Geometry check sheet. Reference: the model listing, model coordinates, mm. A direction names the side the tool comes from. Round coordinates to 2 decimals unless told otherwise and drop trailing zeros. Order: outer loops, then holes, each group sorted by start corner. A loop starts at its lowest first (then second) coordinate and runs counter-clockwise, first axis right, second up. Notation, with made-up numbers: (83, 59) - (120, 59) arc R7 cw to (120, 66) - close; hole circle Ø3 at (-9, 49). An arc over 180 degrees is marked (long way). Use a Markdown table: item, result. Add a question column.
(1) Thickness scan on line 1 along Z through (x, y) = (12.25, -9.5); line 2 along Y through (x, z) = (6, 10.25); line 3 along X through (y, z) = (9, 3.75). Record the ranges inside material, lowest first. Write a range as [from, to].
(2) Access from +Z, -Z, +X, -X, +Y, -Y to the whole of each face (thin tool, end or side, straight path). Record for faces 4 (the face through (8.3, -22, 0.5)), 5 (the face through (0, 16.5, 7)), 6 (the face through (12, 0, 3.54)).
(3) Mould release check, pull along Z, two halves, no side actions. Record for faces 1 (the face through (12.085, -12.692, 8.977)), 2 (the face through (0, 20, 1)), 3 (the face through (13.2, 0, 9)): released by +Z, released by -Z, zero draft, split by the parting line, or undercut.
(4) Section check D-D on z = 9. Record the boundary of the cut face in (x, y).
(5) Section check A-A on x = 11.75. Record the boundary of the cut face in (y, z).
(6) Section check B-B on y = 7.5. Record the boundary of the cut face in (x, z), then the cut area to 3 significant figures.
(7) Gauge pin test, flat ends, axial feed: P1, Ø1.8, axis at x = 12.5, y = -5, coming from the +Z side; P2, Ø4, axis at y = -18.5, z = 2, coming from the +X side; P3, Ø3.5, axis at x = -5.5, z = 5.5, coming from the +Y side. Record the tip position at first contact, or that the pin passes through.
(8) Section check C-C on x = 7.5. Record the boundary of the cut face in (y, z), then the cut area to 3 significant figures.
```python
from build123d import *

# Parameters (mm, degrees)
SKETCH_1_W          = 22
SKETCH_1_H          = 53
EXTRUDE_1_DEPTH     = 1
CUT_EXTRUDE_1_DEPTH = 29.70975444
SKETCH_3_W          = 22
SKETCH_3_H          = 33
EXTRUDE_2_DEPTH     = 12
EXTRUDE_3_DEPTH     = 2.2
CHAMFER_1_SIZE      = 7
FILLET_1_R          = 5


with BuildPart() as part:
    # 草图1 → 凸台-拉伸1 (new body)
    with BuildSketch(Plane.XY):
        Rectangle(SKETCH_1_W, SKETCH_1_H)
    extrude(amount=EXTRUDE_1_DEPTH)

    # 草图2 → 切除-拉伸1 (cut, through all)
    with BuildSketch(Plane.XY.offset(1)):
        with BuildLine():
            Line((1.5, 24), (6.3, 24))
            ThreePointArc((6.3, 24), (8.3, 22), (6.3, 20))
            Line((6.3, 20), (1.5, 20))
            ThreePointArc((1.5, 20), (-0.5, 22), (1.5, 24))
        make_face()
    cut_extrude_1 = extrude(amount=-CUT_EXTRUDE_1_DEPTH, mode=Mode.SUBTRACT)

    # 镜向1: 切除-拉伸1 across plane
    add(cut_extrude_1.mirror(Plane.ZX), mode=Mode.SUBTRACT)

    # 草图3 → 凸台-拉伸2 (add)
    with BuildSketch(Plane.XY.offset(1)):
        Rectangle(SKETCH_3_W, SKETCH_3_H)
    extrude(amount=EXTRUDE_2_DEPTH)

    # 草图4 → 凸台-拉伸3 (add)
    with BuildSketch(Plane(origin=(11, 0, 0), x_dir=(0, 0, -1), z_dir=(1, 0, 0))):
        with BuildLine():
            Line((-10.054063842, -11.63862159), (-10.054063842, 11.63862159))
            ThreePointArc((-10.054063842, 11.63862159), (-9, 12.692685432), (-7.945936158, 11.63862159))
            Line((-7.945936158, 11.63862159), (-7.945936158, -11.63862159))
            ThreePointArc((-7.945936158, -11.63862159), (-9, -12.692685432), (-10.054063842, -11.63862159))
        make_face()
        with BuildLine():
            Line((-1.432333752, -11.63862159), (-1.432333752, 11.63862159))
            ThreePointArc((-1.432333752, 11.63862159), (-2.486397594, 12.692685432), (-3.540461436, 11.63862159))
            Line((-3.540461436, 11.63862159), (-3.540461436, -11.63862159))
            ThreePointArc((-3.540461436, -11.63862159), (-2.486397594, -12.692685432), (-1.432333752, -11.63862159))
        make_face()
    extrude(amount=EXTRUDE_3_DEPTH)

    # 倒角1
    chamfer_1_edges = [part.edges().sort_by_distance(p)[0] for p in [
        (-11, -26.5, 0.5),
        (-11, 26.5, 0.5),
    ]]
    chamfer(chamfer_1_edges, length=CHAMFER_1_SIZE)

    # 圆角1
    fillet_1_edges = [part.edges().sort_by_distance(p)[0] for p in [
        (11, -26.5, 0.5),
        (11, 26.5, 0.5),
    ]]
    fillet(fillet_1_edges, radius=FILLET_1_R)


solid = part.part
```
Check sheet entries:
| question | item | result |
|---|---|---|
| 1 | line 1 | z = [1.43, 3.54], [7.95, 10.05] |
| 1 | line 2 | y = [-16.5, 16.5] |
| 1 | line 3 | x = [-11, 11] |
| 2 | face 4 | +Z, -Z |
| 2 | face 5 | +Z, +X, -X, +Y |
| 2 | face 6 | +X, +Y, -Y |
| 3 | face 1 | undercut |
| 3 | face 2 | released by +Z |
| 3 | face 3 | zero draft |
| 4 | outline | (-11, -16.5) - (11, -16.5) - (11, -12.69) - (13.2, -12.69) - (13.2, 12.69) - (11, 12.69) - (11, 16.5) - (-11, 16.5) - close |
| 5 | outline | (-11.64, 1.43) - (11.64, 1.43) arc R1.05 ccw to (11.64, 3.54) - (-11.64, 3.54) arc R1.05 ccw to start; (-11.64, 7.95) - (11.64, 7.95) arc R1.05 ccw to (11.64, 10.05) - (-11.64, 10.05) arc R1.05 ccw to start |
| 6 | outline | (-11, 0) - (11, 0) - (11, 1.43) - (13.2, 1.43) - (13.2, 3.54) - (11, 3.54) - (11, 7.95) - (13.2, 7.95) - (13.2, 10.05) - (11, 10.05) - (11, 13) - (-11, 13) - close |
| 6 | area | 295 mm2 |
| 7 | P1 | stops at z = 10.05 |
| 7 | P2 | stops at x = 11 |
| 7 | P3 | stops at y = 16.5 |
| 8 | outline | (-26.27, 0) - (-23.6, 0) - (-23.6, 1) - (-26.27, 1) - close; (-20.4, 0) - (20.4, 0) - (20.4, 1) - (16.5, 1) - (16.5, 13) - (-16.5, 13) - (-16.5, 1) - (-20.4, 1) - close; (23.6, 0) - (26.27, 0) - (26.27, 1) - (23.6, 1) - close |
| 8 | area | 442 mm2 |
